Input: part model. Units: mm. Frame: model coordinates. A direction names the side the tool comes from. Give positions to 0.01 mm unless a question says otherwise; leave off trailing zeros. Loops run counter-clockwise (first coordinate to the right, second up) from the corner with the lowest first, then second, coordinate; pieces in that order, holes last. Notation, with made-up numbers: (57.5, 20) - (90.5, 20) arc R20 ccw to (90.5, 44) - close; hole circle Ø1 at (41, -2). An arc over 180 degrees is marked (long way). Answer as a JSON object with one key per item and string values. Group by question number.
(1) Section query B-B (y = 30). Return loops of the section in (x, z), plus the area to 3 significant figures.
(2) Section query A-A (x = 0). Return loops of the section in (y, z).
(3) Access query for faces 5 (the flat face through (67.84, 0, -10)), 6 (the cylindrical face through (61.1, 5.6, 17.3)), 7 (the flat face through (-67.84, 0, -10)), 8 (the flat face through (-1, 0, -20.4)). Directions: +Z, -Z, +X, -X, +Y, -Y. A direction counts if a zero-diameter tool reaches every point of the face in a straight line with its end or side. Return the directions, or none.
(4) Pin query (flat end, axial travel): P1, Ø8, axis at x = 43.5, y = 5.5, coming from the +Z side; P2, Ø5, axis at x = -45, z = -9, coming from the +Y side; P3, Ø5.5, axis at y = -0.5, z = -7, coming from the -X side; P4, Ø8, axis at x = 50, z = 19, coming from the +Y side. Return the tip coordinate at first contact, or that it passes through.
(5) Mould query, pull axis Y, two halves, no side actions, for faces 1 (the flat face through (58, 5, 30)), 2 (the cylindrical face through (-2.75, 17.6, 2.46)), 3 (the flat face through (1, -2.502, -8)), 4 (the flat face through (-1, 2.498, -10)). Classes: +Y half, -Y half, draft (parallel to the pull), parting line (faces both ways), or undercut.
(6) Section query C-C (x = 47). Return loops of the section in (y, z), plus the area to 3 significant figures.
(7) Material intervals for L1, parallel to Y at x = 0, z = 3.7; L2, parallel to Z at x = -2.5, y = 50; L3, parallel to Y at x = -28, z = -15, sorted ascending.
(8) Section query D-D (z = -13.5). Return loops of the section in (x, y).
```python
from build123d import *

# Parameters (mm, degrees)
CROQUIS1_R              = 12.7
SALIENTE_EXTRUIR1_DEPTH = 5
CROQUIS3_W              = 135.679587796
CROQUIS3_H              = 5
SALIENTE_EXTRUIR3_DEPTH = 25.4
CROQUIS4_R              = 3.175
SALIENTE_EXTRUIR4_DEPTH = 25
SALIENTE_EXTRUIR5_DEPTH = 5


with BuildPart() as part:
    # Croquis1 → Saliente-Extruir1 (new body)
    with BuildSketch(Plane.XY):
        Polygon((67.839793898, 2.498030194), (34.641016151, 60), (-34.641016151, 60), (-67.839793898, 2.498030194), align=None)
        with Locations((0, 30)):
            Circle(CROQUIS1_R, mode=Mode.SUBTRACT)
    extrude(amount=SALIENTE_EXTRUIR1_DEPTH)

    # Croquis3 → Saliente-Extruir3 (add)
    with BuildSketch(Plane.XY.offset(5)):
        with Locations((0, -0.001969806)):
            Rectangle(CROQUIS3_W, CROQUIS3_H)
    extrude(amount=-SALIENTE_EXTRUIR3_DEPTH)

    # Croquis4 → Saliente-Extruir4 (add)
    with BuildSketch(Plane.XY.offset(5)):
        with Locations((58.069793898, 4.658030194)):
            Circle(CROQUIS4_R)
    extrude(amount=SALIENTE_EXTRUIR4_DEPTH)

    # Croquis5 → Saliente-Extruir5 (add)
    with BuildSketch(Plane.XY.offset(5)):
        Polygon((70.641016151, 60), (70.641016151, -2.501969806), (67.839793898, -2.501969806), (67.839793898, 2.498030194), (34.641016151, 60), align=None)
        Polygon((-67.839793898, -2.501969806), (-67.839793898, 2.498030194), (-34.641016151, 60), (-70.641016151, 60), (-70.641016151, -2.501969806), align=None)
    extrude(amount=-SALIENTE_EXTRUIR5_DEPTH)


solid = part.part
```
Recorded:
{
 "1": {"outline": "(-70.64, 0) - (-12.7, 0) - (-12.7, 5) - (-70.64, 5) - close; (12.7, 0) - (70.64, 0) - (70.64, 5) - (12.7, 5) - close", "area": "579 mm^2"},
 "2": {"outline": "(-2.5, -20.4) - (2.5, -20.4) - (2.5, 0) - (17.3, 0) - (17.3, 5) - (-2.5, 5) - close; (42.7, 0) - (60, 0) - (60, 5) - (42.7, 5) - close"},
 "3": {"face 5": "-Z, +X, +Y, -Y", "face 6": "+Z", "face 7": "-Z, -X, +Y, -Y", "face 8": "-Z, +X, -X, +Y, -Y"},
 "4": {"P1": "stops at z = 5", "P2": "stops at y = 2.5", "P3": "stops at x = -67.84", "P4": "passes through"},
 "5": {"face 1": "draft", "face 2": "undercut", "face 3": "-Y half", "face 4": "+Y half"},
 "6": {"outline": "(-2.5, -20.4) - (2.5, -20.4) - (2.5, 0) - (60, 0) - (60, 5) - (-2.5, 5) - close", "area": "415 mm^2"},
 "7": {"L1": "y = -2.5 to 17.3, 42.7 to 60", "L2": "z = 0 to 5", "L3": "y = -2.5 to 2.5"},
 "8": {"outline": "(-67.84, -2.5) - (67.84, -2.5) - (67.84, 2.5) - (-67.84, 2.5) - close"}
}
